Autodesk Inventor part; units mm, degrees
ref_plane "body_to_diffuser_kk23_XY" through (-11.8872, 0, 0) normal (1, 0, 0) x (0, 0, -1)
ref_plane "body_to_diffuser_kk23_YZ" through (-11.8872, 0, 0) normal (0, 0, -1) x (0, 1, 0)
ref_plane "body_to_diffuser_kk23_ZX" through (-11.8872, 0, 0) normal (0, 1, 0) x (1, 0, 0)
sketch "Sketch_11" plane through (1.016, 0, 0) normal (1, 0, 0) x (0, 0, -1)
  line L0 (-9.4996, 9.4996) -> (-9.4996, -9.4996)
  line L1 (-9.4996, -9.4996) -> (9.4996, -9.4996)
  line L2 (9.4996, -9.4996) -> (9.4996, 9.4996)
  line L3 (9.4996, 9.4996) -> (-9.4996, 9.4996)
extrude "Extrusion1" add sketch "Sketch_11" against normal blind 15.494
sketch "Sketch_12" plane through (0, 0, 0) normal (0, 0, 1) x (1, 0, 0)
  line L0 (-20.32, 12.8016) -> (-20.32, -12.8016)
  line L1 (-20.32, -12.8016) -> (1.016, -12.8016)
  line L2 (1.016, -12.8016) -> (1.016, -7.9756)
  line L3 (1.016, -7.9756) -> (-13.081, -7.9756)
  line L4 (-13.081, -7.9756) -> (-13.081, -9.4996)
  line L5 (-13.081, -9.4996) -> (-13.335, -9.4996)
  line L6 (-13.335, -9.4996) -> (-14.478, -8.3566)
  line L7 (-14.478, -8.3566) -> (-14.478, 8.3566)
  line L8 (-14.478, 8.3566) -> (-13.335, 9.4996)
  line L9 (-13.335, 9.4996) -> (-13.081, 9.4996)
  line L10 (-13.081, 9.4996) -> (-13.081, 7.9756)
  line L11 (-13.081, 7.9756) -> (1.016, 7.9756)
  line L12 (1.016, 7.9756) -> (1.016, 12.8016)
  line L13 (1.016, 12.8016) -> (-20.32, 12.8016)
extrude "Extrusion2" cut sketch "Sketch_12" along normal mid plane 18.9992
sketch "Sketch_13" plane through (0, 0, 0) normal (0, 1, 0) x (-1, 0, 0)
  line L0 (20.32, -12.8016) -> (20.32, 12.8016)
  line L1 (20.32, 12.8016) -> (-1.016, 12.8016)
  line L2 (-1.016, 12.8016) -> (-1.016, 7.9756)
  line L3 (-1.016, 7.9756) -> (13.081, 7.9756)
  line L4 (13.081, 7.9756) -> (13.081, 9.4996)
  line L5 (13.081, 9.4996) -> (13.335, 9.4996)
  line L6 (13.335, 9.4996) -> (14.478, 8.3566)
  line L7 (14.478, 8.3566) -> (14.478, -8.3566)
  line L8 (14.478, -8.3566) -> (13.335, -9.4996)
  line L9 (13.335, -9.4996) -> (13.081, -9.4996)
  line L10 (13.081, -9.4996) -> (13.081, -7.9756)
  line L11 (13.081, -7.9756) -> (-1.016, -7.9756)
  line L12 (-1.016, -7.9756) -> (-1.016, -12.8016)
  line L13 (-1.016, -12.8016) -> (20.32, -12.8016)
extrude "Extrusion3" cut sketch "Sketch_13" along normal mid plane 18.9992
sketch "Sketch_14" plane through (1.016, 0, 0) normal (1, 0, 0) x (0, 0, -1)
  line L0 (-7.112, -7.112) -> (-1.9812, -7.112)
  line L1 (-1.9812, -7.112) -> (-1.9812, -7.366)
  line L2 (-1.9812, -7.366) -> (1.9812, -7.366)
  line L3 (1.9812, -7.366) -> (1.9812, -7.112)
  line L4 (1.9812, -7.112) -> (7.112, -7.112)
  line L5 (7.112, -7.112) -> (7.112, 7.112)
  line L6 (7.112, 7.112) -> (-7.112, 7.112)
  line L7 (-7.112, 7.112) -> (-7.112, -7.112)
extrude "Extrusion4" cut sketch "Sketch_14" against normal blind 0.762
sketch "Sketch_15" plane through (0, 0, 7.9756) normal (0, 0, 1) x (1, 0, 0)
  line L0 (0.8128, 5.9436) -> (0.8128, 1.524)
  line L1 (0.8128, 1.524) -> (1.016, 1.524)
  line L2 (1.016, 1.524) -> (1.016, 5.9436)
  line L3 (1.016, 5.9436) -> (0.8128, 5.9436)
extrude "Extrusion5" cut sketch "Sketch_15" against normal blind 15.9512
sketch "Sketch_16" plane through (0, 0, 7.9756) normal (0, 0, 1) x (1, 0, 0)
  line L0 (0.8128, -5.9436) -> (1.016, -5.9436)
  line L1 (1.016, -5.9436) -> (1.016, -1.524)
  line L2 (1.016, -1.524) -> (0.8128, -1.524)
  line L3 (0.8128, -1.524) -> (0.8128, -5.9436)
extrude "Extrusion6" cut sketch "Sketch_16" against normal blind 15.9512
sketch "Sketch_17" plane through (0, 7.9756, 0) normal (0, 1, 0) x (1, 0, 0)
  line L0 (0.8128, 5.9436) -> (0.8128, -5.9436)
  line L1 (0.8128, -5.9436) -> (1.016, -5.9436)
  line L2 (1.016, -5.9436) -> (1.016, 5.9436)
  line L3 (1.016, 5.9436) -> (0.8128, 5.9436)
extrude "Extrusion7" cut sketch "Sketch_17" against normal blind 15.9512
sketch "Sketch_48" plane through (0, 0, 7.9756) normal (0, 0, 1) x (1, 0, 0)
  line L0 (-8.3185, 7.9756) -> (-8.3185, 2.8956)
  line L1 (-8.3185, 2.8956) -> (-4.7625, 2.8956)
  line L2 (-4.7625, 2.8956) -> (-4.7625, 7.9756)
  line L3 (-4.7625, 7.9756) -> (-8.3185, 7.9756)
  line L4 (-7.0485, 6.1976) -> (-7.0485, 4.6736)
  line L5 (-7.0485, 4.6736) -> (-6.0325, 4.6736)
  line L6 (-6.0325, 4.6736) -> (-6.0325, 6.1976)
  line L7 (-6.0325, 6.1976) -> (-7.0485, 6.1976)
extrude "Extrusion8" cut sketch "Sketch_48" against normal blind 0.254
sketch "Sketch_50" plane through (0, 0, 7.9756) normal (0, 0, 1) x (1, 0, 0)
  line L0 (-8.3185, -7.9756) -> (-4.7625, -7.9756)
  line L1 (-4.7625, -7.9756) -> (-4.7625, -2.8956)
  line L2 (-4.7625, -2.8956) -> (-8.3185, -2.8956)
  line L3 (-8.3185, -2.8956) -> (-8.3185, -7.9756)
  line L4 (-7.0485, -6.1976) -> (-6.0325, -6.1976)
  line L5 (-6.0325, -6.1976) -> (-6.0325, -4.6736)
  line L6 (-6.0325, -4.6736) -> (-7.0485, -4.6736)
  line L7 (-7.0485, -4.6736) -> (-7.0485, -6.1976)
extrude "Extrusion9" cut sketch "Sketch_50" against normal blind 0.254
sketch "Sketch_51" plane through (0, 0, -7.9756) normal (0, 0, 1) x (1, 0, 0)
  line L0 (-8.3185, 7.9756) -> (-8.3185, 2.8956)
  line L1 (-8.3185, 2.8956) -> (-4.7625, 2.8956)
  line L2 (-4.7625, 2.8956) -> (-4.7625, 7.9756)
  line L3 (-4.7625, 7.9756) -> (-8.3185, 7.9756)
  line L4 (-7.0485, 6.1976) -> (-7.0485, 4.6736)
  line L5 (-7.0485, 4.6736) -> (-6.0325, 4.6736)
  line L6 (-6.0325, 4.6736) -> (-6.0325, 6.1976)
  line L7 (-6.0325, 6.1976) -> (-7.0485, 6.1976)
extrude "Extrusion10" cut sketch "Sketch_51" along normal blind 0.254
sketch "Sketch_52" plane through (0, 0, -7.9756) normal (0, 0, 1) x (1, 0, 0)
  line L0 (-8.3185, -7.9756) -> (-4.7625, -7.9756)
  line L1 (-4.7625, -7.9756) -> (-4.7625, -2.8956)
  line L2 (-4.7625, -2.8956) -> (-8.3185, -2.8956)
  line L3 (-8.3185, -2.8956) -> (-8.3185, -7.9756)
  line L4 (-7.0485, -6.1976) -> (-6.0325, -6.1976)
  line L5 (-6.0325, -6.1976) -> (-6.0325, -4.6736)
  line L6 (-6.0325, -4.6736) -> (-7.0485, -4.6736)
  line L7 (-7.0485, -4.6736) -> (-7.0485, -6.1976)
extrude "Extrusion11" cut sketch "Sketch_52" along normal blind 0.254
sketch "Sketch_21" plane through (-14.478, 0, 0) normal (1, 0, 0) x (0, 0, -1)
  line L0 (-7.5057, -7.5057) -> (7.5057, -7.5057)
  line L1 (7.5057, -7.5057) -> (7.5057, 7.5057)
  line L2 (7.5057, 7.5057) -> (-7.5057, 7.5057)
  line L3 (-7.5057, 7.5057) -> (-7.5057, -7.5057)
extrude "Extrusion12" cut sketch "Sketch_21" along normal blind 5.0038
ref_plane "body_to_diffuser_kk23_XY" through (-11.8872, 0, 0) normal (1, 0, 0) x (0, 0, -1)
ref_plane "body_to_diffuser_kk23_YZ" through (-11.8872, 0, 0) normal (0, 0, -1) x (0, 1, 0)
ref_plane "body_to_diffuser_kk23_ZX" through (-11.8872, 0, 0) normal (0, 1, 0) x (1, 0, 0)
ref_plane "body_to_metal_XY" through (-0.508, 0, 0) normal (-1, 0, 0) x (0, 0, -1)
ref_plane "body_to_metal_YZ" through (-0.508, 0, 0) normal (0, 0, -1) x (0, -1, 0)
ref_plane "body_to_metal_ZX" through (-0.508, 0, 0) normal (0, -1, 0) x (-1, 0, 0)
ref_plane "body_to_pole_XY" through (-0.508, 0, 0) normal (-1, 0, 0) x (0, 0, -1)
ref_plane "body_to_pole_YZ" through (-0.508, 0, 0) normal (0, 0, -1) x (0, -1, 0)
ref_plane "body_to_pole_ZX" through (-0.508, 0, 0) normal (0, -1, 0) x (-1, 0, 0)
properties part number "UB216KKW015C-NR"
Can you work these out from the model? Positions are in its coordinate system, mm. A direction names the side the tool comes from. Give positions to 0.01 mm unless a question says otherwise; leave off trailing zeros. Order: outer loops, then holes, each group sorted by start corner. A loop starts at its lowest first (then second) coordinate and runs counter-clockwise, first axis right, second up. Notation, with made-up numbers: M 35.25,37.25 L 41.25,37.25 A25 ccw 41.25,57.25 Z; hole C -19.75,19.25 d4. An arc over 180 degrees is marked long. Write item = value, one per line. Start each with the question number.
Q1. Will these pins go through, and if not, where does the flat tip stop? pin 1 Ø4 at (x, z) = (-5.5, 1) entering from +Y; pin 2 Ø4 at (y, z) = (1, 0.5) entering from +X; pin 3 Ø5 at (x, y) = (-10.5, -0.5) entering from -Z; pin 4 Ø2 at (x, z) = (-12.5, -2) entering from +Y.
Q2. We'd pull the mould along Y, two halves only. Please class faces 5 (the flat face through (0.254, 0, 0)), 6 (the flat face through (1.016, 0, 7.5)): pulls with the +Y half, pulls with the -Y half, needs draft (parallel to the pull), parting line crosses it, or undercut.
Q3. Suppose I cut it at A-A (x = -11.75). Write out the boundary of the cut face in (y, z), plus the area to 3 significant figures.
Q4. For faces 1 (the flat face through (-12, 0, 7.506)), 2 (the flat face through (-6, 0, 7.976)), 3 (the flat face through (-6.5, 5.4, -7.976)), 4 (the flat face through (0.813, -7.54, -0.08)), which set-ups out of +Z, -Z, +X, -X, +Y, -Y let a thin tool reach every point of the face, with its end or its side?
Q5. I need wall thicknesses on probe 1 along Y at (x, z) = (-12.25, 6.75); probe 2 along Y at (x, z) = (-13.25, -6.75). Which ranges of each line are inside material? Lowest first, please. Write a range as [from, to].
Q6. Suppose I cut it at D-D (x = -5.75). Write out the boundary of the cut face in (y, z).
Q7. Suppose I cut it at B-B (y = 2). Write out the boundary of the cut face in (x, z) (3 decimals), plus the area to 3 significant figures.
Check result:
q1.pin_1 = 7.98
q1.pin_2 = 0.25
q1.pin_3 = -7.98
q1.pin_4 = 9.5
q2.face_5 = undercut
q2.face_6 = needs draft
q3.outline = M -7.98,-7.98 L 7.98,-7.98 L 7.98,7.98 L -7.98,7.98 Z; hole M -7.51,-7.51 L 7.51,-7.51 L 7.51,7.51 L -7.51,7.51 Z
q3.area = 29.1 mm2
q4.face_1 = -X
q4.face_2 = +Z, +X, +Y, -Y
q4.face_3 = -Z, +X, +Y, -Y
q4.face_4 = +X, +Y, -Y
q5.probe_1 = [-7.98, -7.51], [7.51, 7.98]
q5.probe_2 = [-9.5, -7.51], [7.51, 9.5]
q6.outline = M -7.98,-7.72 L -2.9,-7.72 L -2.9,-7.98 L 2.9,-7.98 L 2.9,-7.72 L 7.98,-7.72 L 7.98,7.72 L 2.9,7.72 L 2.9,7.98 L -2.9,7.98 L -2.9,7.72 L -7.98,7.72 Z
q7.outline = M -14.478,-8.357 L -13.335,-9.5 L -13.081,-9.5 L -13.081,-7.976 L 0.813,-7.976 L 0.813,-7.112 L 0.254,-7.112 L 0.254,7.112 L 0.813,7.112 L 0.813,7.976 L -13.081,7.976 L -13.081,9.5 L -13.335,9.5 L -14.478,8.357 L -14.478,7.506 L -9.474,7.506 L -9.474,-7.506 L -14.478,-7.506 Z
q7.area = 164 mm2
